Verification items for the finished model (mm, model axes). A direction names the side the tool comes from. Coordinates: 2 decimals unless noted, no trailing zeros. Order: outer loops, then holes, each group sorted by start corner. A loop starts at its lowest first (then second) coordinate and runs counter-clockwise, first axis right, second up. Notation, with made-up numbers: M 20.25,13.5 L 75.25,13.5 A30 cw 75.25,38.5 Z; hole C 24,80 d9. An arc over 180 degrees is marked long. Answer as a JSON object with one key per item and string values. Group by question number.
(1) Cross-section at C-C (y = 2). Enter the section's corners in (x, z), plus the area to 3 significant figures.
(2) Cross-section at A-A (x = 0). Count the separate pieces of the cut face and the enclosed holes in it, plus the area to 3 significant figures.
(3) Cross-section at B-B (z = 0). Enter the section's corners in (x, y) (3 decimals).
(4) Gauge pin test, flat ends, axial feed: pin 1 Ø8 at (x, z) = (-21, 25) entering from -Y; pin 2 Ø3 at (x, z) = (-10, 10) entering from +Y; pin 3 Ø8 at (y, z) = (7.5, 17.5) entering from +X. Record the tip position at first contact, or that the pin passes through.
(5) Cross-section at D-D (y = 11). Enter the section's corners in (x, z) (3 decimals), plus the area to 3 significant figures.
(6) Mould release check, pull along X, two halves, no side actions. Record for faces 4 (the face through (4, 0, 0)), 5 (the face through (21.39, 11.2, -13.67)), 6 (the face through (-9.76, 11.3, 31)), 7 (the face through (-20.45, 11.2, 12.45)): released by +X, released by -X, zero draft, split by the parting line, or undercut.
(7) Material ranges on line 1 (Z direction, x = -10, y = 3.5); line 2 (X direction, y = 8.25, z = 0.5); line 3 (Y direction, x = -9, z = 7), recorded low to high.
(8) Access from +Z, -Z, +X, -X, +Y, -Y to the whole of each face (thin tool, end or side, straight path). Record for faces 1 (the face through (0.1, 7.7, 14)), 2 (the face through (0.65, 3.8, -1.01)), 3 (the face through (-0.88, 4.3, -19.98)).
from build123d import *

# Parameters (mm, degrees)
F_2_4_2_4_DURCHMESSER_BOHRUNG1_D = 2.4
KREISMUSTER1_COUNT               = 6
F_2_4_2_4_DURCHMESSER_BOHRUNG2_D = 2.4
FASE1_SIZE                       = 1
FASE2_SIZE                       = 1


with BuildPart() as part:
    # Skizze1 → Rotation1 (revolve)
    with BuildSketch(Plane.XY, mode=Mode.PRIVATE) as rotation1_sk:
        Polygon((0, 0), (20, 0), (20, 7.5), (32.5, 7.5), (32.5, 15), (16.075, 15), (16.075, 8), (14, 8), (14, 7.5), (0, 7.5), align=None)
    revolve(rotation1_sk.sketch.rotate(Axis((0, 0, 0), (0, -1, 0)), 90), axis=Axis((0, 0, 0), (0, -1, 0)))

    # Ø2.4 (2.4) Durchmesser Bohrung1 (through all)
    with Locations(Plane(origin=(0, 15, 0), x_dir=(1, 0, 0), z_dir=(0, 1, 0))):
        with Locations((0, 25)):
            f_2_4_2_4_durchmesser_bohrung1 = Hole(F_2_4_2_4_DURCHMESSER_BOHRUNG1_D / 2)

    # Kreismuster1: Ø2.4 (2.4) Durchmesser Bohrung1 ×6 about axis
    kreismuster1_axis = Axis((0, 0, 0), (0, 1, 0))
    for i in range(1, KREISMUSTER1_COUNT):
        add(f_2_4_2_4_durchmesser_bohrung1.rotate(kreismuster1_axis, i * 360 / KREISMUSTER1_COUNT), mode=Mode.SUBTRACT)

    # Ø2.4 (2.4) Durchmesser Bohrung2 (through all)
    with Locations(Plane(origin=(0, 0, 0), x_dir=(-1, 0, 0), z_dir=(0, -1, 0))):
        with Locations((0, 0), (10, 10), (-10, -10), (-10, 10), (10, -10)):
            Hole(F_2_4_2_4_DURCHMESSER_BOHRUNG2_D / 2)

    # Fase1
    fase1_edges = [part.edges().sort_by_distance(p)[0] for p in [
        (0, 15, -16.075),
    ]]
    chamfer(fase1_edges, length=FASE1_SIZE)

    # Fase2
    fase2_edges = [part.edges().sort_by_distance(p)[0] for p in [
        (0, 0, -20),
    ]]
    chamfer(fase2_edges, length=FASE2_SIZE)


solid = part.part
Taken from the geometry:
{
 "1": {"outline": "C 0,0 d40; hole C -10,-10 d2.4; hole C -10,10 d2.4; hole C 0,0 d2.4; hole C 10,-10 d2.4; hole C 10,10 d2.4", "area": "1,230 mm²"},
 "2": {"separate pieces": "4", "enclosed holes": "0", "area": "492 mm²"},
 "3": {"outline": "M -32.5,7.5 L -20,7.5 L -20,1 L -19,0 L -1.2,0 L -1.2,7.5 L -14,7.5 L -14,8 L -16.075,8 L -16.075,14 L -17.075,15 L -32.5,15 Z; M 1.2,0 L 19,0 L 20,1 L 20,7.5 L 32.5,7.5 L 32.5,15 L 17.075,15 L 16.075,14 L 16.075,8 L 14,8 L 14,7.5 L 1.2,7.5 Z"},
 "4": {"pin 1": "stops at y = 7.5", "pin 2": "stops at y = 8", "pin 3": "stops at x = 29.56"},
 "5": {"outline": "C 0,0 d65; hole C -21.651,-12.5 d2.4; hole C -21.651,12.5 d2.4; hole C 0,0 d32.15; hole C 0,-25 d2.4; hole C 0,25 d2.4; hole C 21.651,-12.5 d2.4; hole C 21.651,12.5 d2.4", "area": "2,480 mm²"},
 "6": {"face 4": "zero draft", "face 5": "undercut", "face 6": "split by the parting line", "face 7": "undercut"},
 "7": {"line 1": "z = -17.32 to -11.2, -8.8 to 8.8, 11.2 to 17.32", "line 2": "x = -32.5 to -16.07, 16.07 to 32.5", "line 3": "y = 0 to 7.5"},
 "8": {"face 1": "+Y", "face 2": "+Y, -Y", "face 3": "-Y"}
}
